```python
from build123d import *

# Parameters (mm, degrees)
SKETCH_1_W             = 300
SKETCH_1_H             = 300
EXTRUDE_1_DEPTH        = 1600
CUT_EXTRUDE_1_DEPTH    = 1656.294535725
CUT_EXTRUDE_4_DEPTH    = 1656.294535725
SHELL_2_T              = -1.5
EXTRUDE_2_DEPTH        = 1.5
PATTERN_LINEAR_1_COUNT = 3
PATTERN_LINEAR_1_PITCH = 400
EXTRUDE_3_DEPTH        = 1.5
EXTRUDE_4_DEPTH        = 1.5
FILLET_1_R             = 3


with BuildPart() as part:
    # 草图1 → 凸台-拉伸1 (new body)
    with BuildSketch(Plane.XY):
        with Locations((150, 150)):
            Rectangle(SKETCH_1_W, SKETCH_1_H)
    extrude(amount=EXTRUDE_1_DEPTH)

    # 草图7 → 切除-拉伸1 (cut, through all)
    with BuildSketch(Plane.XY.offset(1600)):
        Polygon((300, 260), (150, 0), (300, 0), align=None)
    extrude(amount=-CUT_EXTRUDE_1_DEPTH, mode=Mode.SUBTRACT)

    # 草图11 → 切除-拉伸4 (cut, through all)
    with BuildSketch(Plane.XY.offset(1600)):
        Polygon((0, 300), (0, 0), (60, 0), align=None)
    extrude(amount=-CUT_EXTRUDE_4_DEPTH, mode=Mode.SUBTRACT)

    # 抽壳2
    shell_2_openings = [part.faces().sort_by_distance(p)[0] for p in [
        (225, 130, 800),
        (300, 280, 800),
    ]]
    offset(amount=SHELL_2_T, openings=shell_2_openings, kind=Kind.INTERSECTION)

    # 草图13 → 凸台-拉伸2 (add)
    with BuildSketch(Plane.XY.offset(1200)):
        Polygon((1.829705854, 298.5), (61.229705854, 1.5), (150.865384615, 1.5), (300, 260), (300, 298.5), align=None)
    extrude_2 = extrude(amount=EXTRUDE_2_DEPTH)

    # 阵列(线性)1: 凸台-拉伸2 ×3
    with Locations(*[(0, 0, -i * PATTERN_LINEAR_1_PITCH) for i in range(1, PATTERN_LINEAR_1_COUNT)]):
        add(extrude_2)

    # 草图14 → 凸台-拉伸3 (add)
    with BuildSketch(Plane.XY.offset(1600)):
        Polygon((300, 260), (300, 10), (290, 0), (150, 0), align=None)
    extrude(amount=-EXTRUDE_3_DEPTH)

    # 草图15 → 凸台-拉伸4 (add)
    with BuildSketch(Plane(origin=(0, 0, 0), x_dir=(-1, 0, 0), z_dir=(0, 0, -1))):
        Polygon((-300, 260), (-150.865384615, 1.5), (-290.865384615, 1.5), (-300.831907642, 11.499943964), align=None)
    extrude(amount=-EXTRUDE_4_DEPTH)

    # 圆角1
    fillet_1_edges = [part.edges().sort_by_distance(p)[0] for p in [
        (0, 300, 800),
    ]]
    fillet(fillet_1_edges, radius=FILLET_1_R)


solid = part.part
```
Input: part model. Units: mm. Frame: model coordinates. A direction names the side the tool comes from. Coordinates: 2 decimals unless noted, no trailing zeros. Write each loop counter-clockwise with the first axis right and the second up, starting at its lowest first coordinate (ties: lowest second). Pieces come first, ordered by that corner, then holes.
1) Section B-B on z = 96.5. Output: boundary loops of the cut face in (x, y).
2) Section A-A on x = 198. Output: boundary loops of the cut face in (y, z), and give its area (3 significant figures).
3) Mould query, pull axis Z, two halves, no side actions, for faces 3 (the flat face through (152, 152, 1600)), 4 (the flat face through (149, 185, 400)), 5 (the flat face through (149, 152, 0)), 6 (the flat face through (30.774, 146.131, 811.2)). Classes: pulls with the +Z half, pulls with the -Z half, needs draft (parallel to the pull), parting line crosses it, or undercut.
4) Pin query (flat end, axial travel): pin 1 Ø5 at (x, z) = (103.5, 374) entering from -Y; pin 2 Ø4 at (y, z) = (245.5, 494) entering from +X; pin 3 Ø10 at (y, z) = (72.5, 760.5) entering from +X; pin 4 Ø3 at (y, z) = (127.5, 525) entering from -X. Return the tip coordinate at first contact, or that it passes through.
5) Set-up query: faces 1 (the flat face through (149, 185, 1200)), 2 (the flat face through (90, 0, 804)). Return all of +Z, -Z, +X, -X, +Y, -Y with unobstructed straight access to the full face (end or side cutting, diameter ignored); none if empty.
6) Section C-C on x = 74.5. Output: boundary loops of the cut face in (y, z), and give its area (3 significant figures).
7) Material intervals for line 1 along Z through (x, y) = (227.5, 251.5); line 2 along Y through (x, z) = (93.5, 76); line 3 along Z through (x, y) = (274, 41.5), sorted ascending.
8) Section D-D on y = 178. Output: boundary loops of the cut face in (x, z).
Check result:
1. outline: (0.72, 296.41) - (60, 0) - (150, 0) - (150.87, 1.5) - (61.23, 1.5) - (1.83, 298.5) - (300, 298.5) - (300, 300) - (3.66, 300) arc R3 ccw to start
2. outline: (0, 1598.5) - (298.5, 1598.5) - (298.5, 1201.5) - (83.2, 1201.5) - (83.2, 1200) - (298.5, 1200) - (298.5, 801.5) - (83.2, 801.5) - (83.2, 800) - (298.5, 800) - (298.5, 401.5) - (83.2, 401.5) - (83.2, 400) - (298.5, 400) - (298.5, 1.5) - (1.5, 1.5) - (1.5, 0) - (300, 0) - (300, 1600) - (0, 1600) - close
2. area: 4,260 mm2
3. face 3: pulls with the +Z half
3. face 4: undercut
3. face 5: pulls with the -Z half
3. face 6: needs draft
4. pin 1: stops at y = 0
4. pin 2: stops at x = 12.83
4. pin 3: stops at x = 48.03
4. pin 4: stops at x = 34.2
5. face 1: +X
5. face 2: +Z, -Z, +X, -X, -Y
6. outline: (0, 0) - (300, 0) - (300, 1600) - (0, 1600) - close; hole (1.5, 1.5) - (298.5, 1.5) - (298.5, 400) - (1.5, 400) - close; hole (1.5, 401.5) - (298.5, 401.5) - (298.5, 800) - (1.5, 800) - close; hole (1.5, 801.5) - (298.5, 801.5) - (298.5, 1200) - (1.5, 1200) - close; hole (1.5, 1201.5) - (298.5, 1201.5) - (298.5, 1598.5) - (1.5, 1598.5) - close
6. area: 7,030 mm2
7. line 1: z = 0 to 1.5, 400 to 401.5, 800 to 801.5, 1200 to 1201.5, 1598.5 to 1600
7. line 2: y = 0 to 1.5, 298.5 to 300
7. line 3: z = 0 to 1.5, 1598.5 to 1600
8. outline: (24.4, 0) - (300.27, 0) - (300.27, 1.5) - (25.93, 1.5) - (25.93, 400) - (252.69, 400) - (252.69, 401.5) - (25.93, 401.5) - (25.93, 800) - (252.69, 800) - (252.69, 801.5) - (25.93, 801.5) - (25.93, 1200) - (252.69, 1200) - (252.69, 1201.5) - (25.93, 1201.5) - (25.93, 1598.5) - (300, 1598.5) - (300, 1600) - (24.4, 1600) - close
